```python
from build123d import *
from build123d.topology import SkipClean

# Parameters (mm, degrees)
SKETCH2_W               = 78
SKETCH2_H               = 126
BOSS_EXTRUDE1_DEPTH     = 13
SKETCH3_W               = 126
SKETCH3_H               = 77
BOSS_EXTRUDE2_DEPTH     = 13
FILLET1_R               = 25
SKETCH4_R               = 9
CUT_EXTRUDE1_DEPTH      = 128.647953372
SKETCH5_R               = 25
BOSS_EXTRUDE3_DEPTH     = 38
BOSS_EXTRUDE4_DEPTH     = 25
CUT_EXTRUDE3_DEPTH      = 128.647953372
CUT_EXTRUDE3_DEPTH_BACK = 128.647953372
SKETCH5_5_R             = 16
RIB1_START              = -7.5
RIB1_DEPTH              = 15
SKETCH7_R               = 9
CUT_EXTRUDE4_DEPTH      = 107.85972113


with BuildPart() as part:
    # Sketch2 → Boss-Extrude1 (new body)
    with BuildSketch(Plane(origin=(0, 0, 0), x_dir=(1, 0, 0), z_dir=(0, 1, 0))):
        Rectangle(SKETCH2_W, SKETCH2_H)
    extrude(amount=BOSS_EXTRUDE1_DEPTH)

    # Sketch3 → Boss-Extrude2 (add)
    with BuildSketch(Plane.ZY.offset(39)):
        with Locations((0, 51.5)):
            Rectangle(SKETCH3_W, SKETCH3_H)
    extrude(amount=-BOSS_EXTRUDE2_DEPTH)

    # Fillet1
    fillet1_edges = [part.edges().sort_by_distance(p)[0] for p in [
        (-32.5, 90, -63),
        (-32.5, 90, 63),
    ]]
    fillet(fillet1_edges, radius=FILLET1_R)

    # Sketch4 → Cut-Extrude1 (cut, through all)
    with BuildSketch(Plane(origin=(-26, 0, 0), x_dir=(0, 0, -1), z_dir=(1, 0, 0))):
        with Locations((-44, 65)):
            Circle(SKETCH4_R)
        with Locations((44, 65)):
            Circle(SKETCH4_R)
    extrude(amount=-CUT_EXTRUDE1_DEPTH, mode=Mode.SUBTRACT)

    # Sketch5 → Boss-Extrude3 (add)
    with BuildSketch(Plane(origin=(-26, 0, 0), x_dir=(0, 0, -1), z_dir=(1, 0, 0))):
        with Locations((0, 51)):
            Circle(SKETCH5_R)
    extrude(amount=BOSS_EXTRUDE3_DEPTH)

    # Sketch5<3> → Boss-Extrude4 (add)
    with BuildSketch(Plane(origin=(-26, 0, 0), x_dir=(0, 0, -1), z_dir=(1, 0, 0))):
        with BuildLine():
            Line((-9, 90), (-19, 90))
            Line((-19, 90), (-19, 67.248076809))
            ThreePointArc((-19, 67.248076809), (0, 76), (19, 67.248076809))
            Line((19, 67.248076809), (19, 90))
            Line((19, 90), (9, 90))
            ThreePointArc((9, 90), (0, 81), (-9, 90))
        make_face()
    extrude(amount=BOSS_EXTRUDE4_DEPTH)

    # Sketch5<5> → Cut-Extrude3 (cut, two sides: drawn at the far end of the back side and taken through both)
    with SkipClean():  # the faces are left unmerged after this step: merging them gives an invalid solid
        with BuildSketch(Plane(origin=(-26, 0, 0), x_dir=(0, 0, -1), z_dir=(1, 0, 0)).offset(-CUT_EXTRUDE3_DEPTH_BACK)):
            with Locations((0, 51)):
                Circle(SKETCH5_5_R)
            with BuildLine():
                Line((9, 90), (-9, 90))
                ThreePointArc((-9, 90), (0, 81), (9, 90))
            make_face()
        extrude(amount=CUT_EXTRUDE3_DEPTH + CUT_EXTRUDE3_DEPTH_BACK, mode=Mode.SUBTRACT)
    add(part.part.scale(1), mode=Mode.REPLACE)  # the faces are merged on a copy

    # Rib1: read off the stored shape, not the designer's step
    # Rib1 outline → Rib1 (add)
    with BuildSketch(Plane.XY.offset(RIB1_START)):
        Polygon((12, 26), (12, 27.151519965), (-26, 27.151519965), (-26, 13), (39, 13), align=None)
    extrude(amount=RIB1_DEPTH)

    # Sketch7 → Cut-Extrude4 (cut, symmetric)
    with BuildSketch(Plane(origin=(0, 13, 0), x_dir=(1, 0, 0), z_dir=(0, 1, 0))):
        with Locations(Location((14, 44, 0), (0, 0, 270))):
            Circle(SKETCH7_R)
    cut_extrude4 = extrude(amount=CUT_EXTRUDE4_DEPTH, both=True, mode=Mode.SUBTRACT)

    # Mirror1: Cut-Extrude4 across plane
    add(cut_extrude4.mirror(Plane.XY), mode=Mode.SUBTRACT)


solid = part.part
```
Could you check a few things on this model? Use its own coordinates, in mm. A direction names the side the tool comes from. Round coordinates to 2 decimals unless told otherwise and drop trailing zeros. Order: outer loops, then holes, each group sorted by start corner. A loop starts at its lowest first (then second) coordinate and runs counter-clockwise, first axis right, second up. Notation, with made-up numbers: (-5.75, -29) -> (23.25, -29) arc R26 cw to (23.25, -15) -> close; hole circle Ø7 at (72.5, 56.25). An arc over 180 degrees is marked (long way). One line per question, with ' | ' between items.
Q1. If we section it at C-C on x = -33: Write out the boundary of the cut face in (y, z).
Computed values:
outline: (0, -63) -> (65, -63) arc R25 ccw to (90, -38) -> (90, -9) arc R9 cw to (90, 9) -> (90, 38) arc R25 ccw to (65, 63) -> (0, 63) -> close; hole circle Ø32 at (51, 0); hole circle Ø18 at (65, -44); hole circle Ø18 at (65, 44)
Q2. If I drill on line 1 (Z direction, x = -11, y = 51); line 2 (X direction, y = 7.75, z = 44); line 3 (Z direction, x = 3.5, y = 21), over which ranges is the centre line in solid material (lowest first)? Write a range as from..to.
Computed values:
line 1: -25..-16, 16..25 | line 2: -39..5, 23..39 | line 3: -7.5..7.5
Q3. Which directions (+Z, -Z, +X, -X, +Y, -Y) give clear straight access to the entire face, cutting with the end or side of a thin tool? Please do faces 1 (the face through (12, 67.3, -0.4)), 2 (the face through (6, 13, 35)), 3 (the face through (-26, 43, -42)), 4 (the face through (-18, 10, -63)), 5 (the face through (-14, 79, 19)).
Computed values:
face 1: +Z, -Z, +X, +Y | face 2: +Z, +X | face 3: -Z, +X | face 4: -Z, +X, -X, +Y, -Y | face 5: +Z, +X, +Y
Q4. If we section it at A-A on z = 0: Write out the boundary of the cut face in (x, y).
Computed values:
outline: (-39, 0) -> (39, 0) -> (39, 13) -> (12, 26) -> (12, 35) -> (-39, 35) -> close; (-39, 67) -> (12, 67) -> (12, 76) -> (-1, 76) -> (-1, 81) -> (-39, 81) -> close
Q5. If we section it at D-D on z = 44: Write out the boundary of the cut face in (x, y), plus the area to 3 significant figures.
Computed values:
outline: (-39, 0) -> (5, 0) -> (5, 13) -> (-26, 13) -> (-26, 56) -> (-39, 56) -> close; (-39, 74) -> (-26, 74) -> (-26, 89.27) -> (-39, 89.27) -> close; (23, 0) -> (39, 0) -> (39, 13) -> (23, 13) -> close | area: 1,540 mm²
Q6. We'd pull the mould along Y, two halves only. Please class faces 6 (the face through (-1, 20, 7.5)), 7 (the face through (-1, 0, -1)), 8 (the face through (-18, 10, 63)), 9 (the face through (-24, 90, 17)): released by +Y, released by -Y, zero draft, split by the parting line, or undercut.
Computed values:
face 6: undercut | face 7: released by -Y | face 8: zero draft | face 9: released by +Y
Q7. If we section it at B-B on y = 51: Write out the boundary of the cut face in (x, z).
Computed values:
outline: (-39, -63) -> (-26, -63) -> (-26, -25) -> (12, -25) -> (12, -16) -> (-39, -16) -> close; (-39, 16) -> (12, 16) -> (12, 25) -> (-26, 25) -> (-26, 63) -> (-39, 63) -> close
Q8. I'm going to push flat-ended pins straight in: pin 1 (4 mm diameter, centred on x = 1.5, y = 20.5, fed in from +Z); pin 2 (4 mm diameter, centred on x = -7, y = 22, fed in from -Z); pin 3 (1.5 mm diameter, centred on x = 6, y = 57.5, fed in from +Z). Where does each tip first touch, or does it pass through?
Computed values:
pin 1: z = 7.5 | pin 2: z = -7.5 | pin 3: z = 24.33
